Verification items for the finished model (mm, model axes). A direction names the side the tool comes from. Coordinates: 2 decimals unless noted, no trailing zeros. Write each loop counter-clockwise with the first axis right and the second up, starting at its lowest first coordinate (ties: lowest second). Pieces come first, ordered by that corner, then holes. Notation, with made-up numbers: (54, -36.75) -> (88, -36.75) arc R15 cw to (88, -31.75) -> close; hole circle Ø10 at (-22.75, -25.5). An arc over 180 degrees is marked (long way). Write each question's results on one line, items separated by ' | '. Start each with the question number.
from build123d import *

# Parameters (mm, degrees)
F0_W      = 40.5
F0_H      = 20
F1_DEPTH  = 36
F2_R      = 7
F3_DEPTH  = 2
F4_R      = 3
F5_DEPTH  = 4
F6_W      = 18
F6_H      = 2
F7_DEPTH  = 7.5
F8_W      = 18
F8_H      = 2
F9_DEPTH  = 7.5
F10_R     = 2.25
F11_DEPTH = 25
F12_W     = 6
F12_H     = 3
F13_DEPTH = 7
F13_TAPER = 3


with BuildPart() as f1:
    # F0 (on Top) → F1 (new body)
    with BuildSketch(Plane.XY):
        with Locations((-20.25, -10)):
            Rectangle(F0_W, F0_H)
    extrude(amount=F1_DEPTH)

    # F2 (on face) → F3 (join)
    with BuildSketch(Plane.XY.offset(36)):
        with Locations((-10.4, -10)):
            Circle(F2_R)
    extrude(amount=F3_DEPTH)

    # F4 (on face) → F5 (join)
    with BuildSketch(Plane.XY.offset(38)):
        with Locations((-10.4, -10)):
            Circle(F4_R)
    extrude(amount=F5_DEPTH)

    # F6 (on face) → F7 (join)
    with BuildSketch(Plane.YZ):
        with Locations((-10, 27.2)):
            Rectangle(F6_W, F6_H)
    extrude(amount=F7_DEPTH)

    # F8 (on face) → F9 (join)
    with BuildSketch(Plane(origin=(-40.5, 0, 0), x_dir=(0, -1, 0), z_dir=(-1, 0, 0))):
        with Locations((10, 27.2)):
            Rectangle(F8_W, F8_H)
    extrude(amount=F9_DEPTH)

    # F10 (on face) → F11 (cut)
    with BuildSketch(Plane.XY.offset(28.2)):
        with Locations((5, -15)):
            Circle(F10_R)
        with Locations((5, -5)):
            Circle(F10_R)
        with Locations((-45.5, -5)):
            Circle(F10_R)
        with Locations((-45.5, -15)):
            Circle(F10_R)
    extrude(amount=-F11_DEPTH, mode=Mode.SUBTRACT)

    # F12 (on face) → F13 (join)
    with BuildSketch(Plane.YZ):
        with Locations((-10, 2.5268535551)):
            Rectangle(F12_W, F12_H)
    extrude(amount=F13_DEPTH, taper=F13_TAPER)


solid = f1.part
1. Sectioned sample at B-B on y = -5. Record the cut outline in (x, z), plus the area to 3 significant figures.
2. Depth check by flat-ended pin: pin 1 Ø8 at (y, z) = (-14.5, 11.5) entering from -X; pin 2 Ø1.6 at (x, z) = (4, 27) entering from -Y; pin 3 Ø7 at (x, y) = (-45.5, -5) entering from +Z; pin 4 Ø4 at (x, y) = (-45.5, -15) entering from +Z. Enter the tip coordinate at first touch or a pass-through.
3. Tool access check on faces 1 (the flat face through (-7, -10, 38)), 2 (the flat face through (3, -10, 26.2)), 3 (the flat face through (-43, -10, 26.2)), 4 (the flat face through (3, -10, 28.2)). Record the directions out of +Z, -Z, +X, -X, +Y, -Y that give a thin tool (end or side, any length) a straight path to the whole face; none if there is none.
4. Sectioned sample at C-C on x = -10.4. Record the cut outline in (y, z).
5. Sectioned sample at A-A on x = -45.5. Record the cut outline in (y, z), plus the area to 3 significant figures.
6. Mould release check, pull along Z, two halves, no side actions. Record for faces 5 (the flat face through (-43, -10, 28.2)), 6 (the flat face through (0, -10, 18)), 7 (the flat face through (-44, -1, 27)): +Z half, -Z half, draft (parallel to the pull), parting line (faces both ways), or undercut.
7. Material ranges on probe 1 along Y at (x, z) = (5, 27.65); probe 2 along X at (y, z) = (-5.25, 30); probe 3 along Z at (x, y) = (-32, -13.25), recorded low to high. Write a range as from..to.
8. Sectioned sample at D-D on y = -16.25. Record the cut outline in (x, z), plus the area to 3 significant figures.
Computed values:
1) outline: (-48, 26.2) -> (-47.75, 26.2) -> (-47.75, 28.2) -> (-48, 28.2) -> close; (-43.25, 26.2) -> (-40.5, 26.2) -> (-40.5, 0) -> (0, 0) -> (0, 26.2) -> (2.75, 26.2) -> (2.75, 28.2) -> (0, 28.2) -> (0, 36) -> (-5.5, 36) -> (-5.5, 38) -> (-15.3, 38) -> (-15.3, 36) -> (-40.5, 36) -> (-40.5, 28.2) -> (-43.25, 28.2) -> close; (7.25, 26.2) -> (7.5, 26.2) -> (7.5, 28.2) -> (7.25, 28.2) -> close | area: 1,490 mm^2
2) pin 1: stops at x = -40.5 | pin 2: stops at y = -19 | pin 3: stops at z = 28.2 | pin 4: passes through
3) face 1: +Z | face 2: +X, +Y, -Y | face 3: -Z, -X, +Y, -Y | face 4: +Z, +X, +Y, -Y
4) outline: (-20, 0) -> (0, 0) -> (0, 36) -> (-3, 36) -> (-3, 38) -> (-7, 38) -> (-7, 42) -> (-13, 42) -> (-13, 38) -> (-17, 38) -> (-17, 36) -> (-20, 36) -> close
5) outline: (-19, 26.2) -> (-17.25, 26.2) -> (-17.25, 28.2) -> (-19, 28.2) -> close; (-12.75, 26.2) -> (-7.25, 26.2) -> (-7.25, 28.2) -> (-12.75, 28.2) -> close; (-2.75, 26.2) -> (-1, 26.2) -> (-1, 28.2) -> (-2.75, 28.2) -> close | area: 18.0 mm^2
6) face 5: +Z half | face 6: undercut | face 7: draft
7) probe 1: y = -19..-17.25, -12.75..-7.25, -2.75..-1 | probe 2: x = -40.5..0 | probe 3: z = 0..36
8) outline: (-48, 26.2) -> (-47.37, 26.2) -> (-47.37, 28.2) -> (-48, 28.2) -> close; (-43.63, 26.2) -> (-40.5, 26.2) -> (-40.5, 0) -> (0, 0) -> (0, 26.2) -> (3.13, 26.2) -> (3.13, 28.2) -> (0, 28.2) -> (0, 36) -> (-7.25, 36) -> (-7.25, 38) -> (-13.55, 38) -> (-13.55, 36) -> (-40.5, 36) -> (-40.5, 28.2) -> (-43.63, 28.2) -> close; (6.87, 26.2) -> (7.5, 26.2) -> (7.5, 28.2) -> (6.87, 28.2) -> close | area: 1,490 mm^2
